Read the model definition and answer for the solid it produces. Units are mm, in the model's axes. Face numbers are marked on the shaded views. A direction names the side the tool comes from. Round coordinates to 2 decimals unless told otherwise and drop trailing zeros. Write each loop counter-clockwise with the first axis right and the second up, starting at its lowest first coordinate (ties: lowest second). Pieces come first, ordered by that corner, then holes. Notation, with made-up numbers: (-32, 10.25) -> (-10, 10.25) arc R36 ccw to (-10, 47.25) -> close; hole circle Ø3 at (-15, 62.25). An arc over 180 degrees is marked (long way). Return JSON: item names as keys, results as strings.
from build123d import *

# Parameters (mm, degrees)
SKETCH1_W           = 60
SKETCH1_H           = 55
BOSS_EXTRUDE1_DEPTH = 1
SKETCH2_W           = 42
SKETCH2_H           = 9
BOSS_EXTRUDE2_DEPTH = 27
SKETCH3_W           = 13
SKETCH3_H           = 16
BOSS_EXTRUDE3_DEPTH = 12
SKETCH4_W           = 32
SKETCH4_H           = 39
BOSS_EXTRUDE4_DEPTH = 22


with BuildPart() as part:
    # Sketch1 → Boss-Extrude1 (new body)
    with BuildSketch(Plane(origin=(0, 0, 0), x_dir=(1, 0, 0), z_dir=(0, 1, 0))):
        Rectangle(SKETCH1_W, SKETCH1_H)
    extrude(amount=BOSS_EXTRUDE1_DEPTH)

    # Sketch2 → Boss-Extrude2 (add)
    with BuildSketch(Plane(origin=(0, 1, 0), x_dir=(1, 0, 0), z_dir=(0, 1, 0))):
        with Locations((0, 26)):
            Rectangle(SKETCH2_W, SKETCH2_H)
        with Locations((0, -26)):
            Rectangle(SKETCH2_W, SKETCH2_H)
    extrude(amount=BOSS_EXTRUDE2_DEPTH)

    # Sketch3 → Boss-Extrude3 (add)
    with BuildSketch(Plane(origin=(0, 1, 0), x_dir=(1, 0, 0), z_dir=(0, 1, 0))):
        with Locations((-23.5, 0)):
            Rectangle(SKETCH3_W, SKETCH3_H)
        with Locations((23.5, 0)):
            Rectangle(SKETCH3_W, SKETCH3_H)
    extrude(amount=BOSS_EXTRUDE3_DEPTH)

    # Sketch4 → Boss-Extrude4 (add)
    with BuildSketch(Plane(origin=(0, 1, 0), x_dir=(1, 0, 0), z_dir=(0, 1, 0))):
        Rectangle(SKETCH4_W, SKETCH4_H)
    extrude(amount=BOSS_EXTRUDE4_DEPTH)


solid = part.part
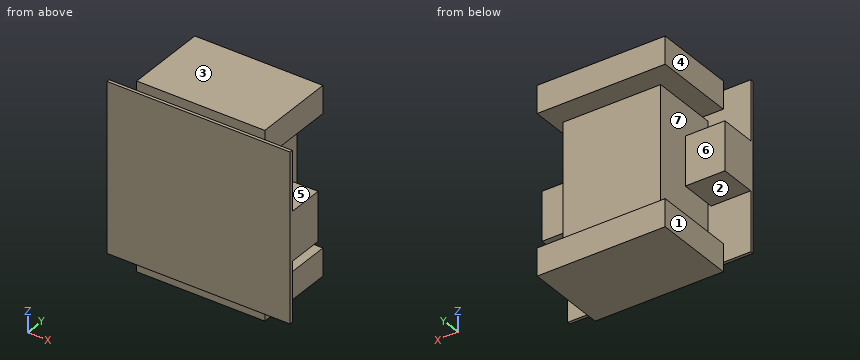
Item 1: Section A-A (y = 3) is taken. Give the vertices of the cut face in (x, z), then the cut area to 3 significant figures.
Worked answers:
{"outline": "(-30, -8) -> (-17, -8) -> (-17, 8) -> (-30, 8) -> close; (-21, -30.5) -> (21, -30.5) -> (21, -21.5) -> (-21, -21.5) -> close; (-21, 21.5) -> (21, 21.5) -> (21, 30.5) -> (-21, 30.5) -> close; (-16, -19.5) -> (16, -19.5) -> (16, 19.5) -> (-16, 19.5) -> close; (17, -8) -> (30, -8) -> (30, 8) -> (17, 8) -> close", "area": "2,420 mm2"}
Item 2: A tool of negligible diameter and unlimited length cuts with its end or side. For the marked faces 4, 5, 6 and 7, from which of +Z, -Z, +X, -X, +Y, -Y can it reach the whole face along a straight path? Write none if from no direction.
Worked answers:
{"face 4": "+Z, -X, +Y", "face 5": "+X, +Y", "face 6": "-X, +Y", "face 7": "+Y"}
Item 3: Section B-B (y = 15.75) is taken. Give the vertices of the cut face in (x, z).
Worked answers:
{"outline": "(-21, -30.5) -> (21, -30.5) -> (21, -21.5) -> (-21, -21.5) -> close; (-21, 21.5) -> (21, 21.5) -> (21, 30.5) -> (-21, 30.5) -> close; (-16, -19.5) -> (16, -19.5) -> (16, 19.5) -> (-16, 19.5) -> close"}
Item 4: Straight lines are drawn through the part: L1, parallel to Z at x = 6.5, y = 15.5; L2, parallel to Z at x = -18.5, y = 5.5; L3, parallel to X at y = 2, z = -4.5. For each, find the intervals that lie inside material, in ascending order. Write a range as [from, to].
Worked answers:
{"L1": "z = [-30.5, -21.5], [-19.5, 19.5], [21.5, 30.5]", "L2": "z = [-30.5, -21.5], [-8, 8], [21.5, 30.5]", "L3": "x = [-30, -17], [-16, 16], [17, 30]"}
Item 5: For a pull along Z with two mould halves and no side action, classify the marked faces 1, 2 and 3 as released by +Z, released by -Z, zero draft, split by the parting line, or undercut.
Worked answers:
{"face 1": "zero draft", "face 2": "undercut", "face 3": "released by +Z"}
Item 6: Section C-C (x = -5.5) is taken. Give the vertices of the cut face in (y, z).
Worked answers:
{"outline": "(0, -27.5) -> (1, -27.5) -> (1, -30.5) -> (28, -30.5) -> (28, -21.5) -> (1, -21.5) -> (1, -19.5) -> (23, -19.5) -> (23, 19.5) -> (1, 19.5) -> (1, 21.5) -> (28, 21.5) -> (28, 30.5) -> (1, 30.5) -> (1, 27.5) -> (0, 27.5) -> close"}
Item 7: Flat-ended cylindrical pins translate along their axes: pin 1 (6 mm diameter, centred on y = 16.5, z = 20, fed in from +X); pin 2 (5 mm diameter, centred on y = 19, z = -14, fed in from -X); pin 3 (7 mm diameter, centred on y = 8.5, z = 28, fed in from -X). Find the tip coordinate at first contact, or state that the pin passes through.
Worked answers:
{"pin 1": "stops at x = 21", "pin 2": "stops at x = -16", "pin 3": "stops at x = -21"}
Item 8: Section D-D (z = 23) is taken. Give the vertices of the cut face in (x, y).
Worked answers:
{"outline": "(-30, 0) -> (30, 0) -> (30, 1) -> (21, 1) -> (21, 28) -> (-21, 28) -> (-21, 1) -> (-30, 1) -> close"}
